Solid Edge part; units mm, degrees
sketch "Sketch1" plane through (0, 0, 0) normal (0, 0, 1) x (1, 0, 0)
  line L0 (8.65, -8) -> (-8.65, -8)
  line L1 (-8.65, -8) -> (-8.65, 8)
  line L2 (-8.65, 8) -> (8.65, 8)
  line L3 (8.65, 8) -> (8.65, -8)
  dimension "D1" = 8.65
  dimension "D2" = 8.65
extrude "Protrusion1" add sketch "Sketch1" along normal blind 6.5
sketch "Sketch2" plane through (0, 0, 6.5) normal (0, 0, 1) x (0, 1, 0)
  circle A0 centre (0, 0.35) radius 4.5
extrude "ExtrudedProtrusion_2" add sketch "Sketch2" along normal blind 7
sketch "Sketch3" plane through (0, 0, 6.5) normal (0, 0, 1) x (1, 0, 0)
  line L0 (8.65, 2) -> (12.15, 2)
  line L1 (12.15, 2) -> (12.15, -2)
  line L2 (12.15, -2) -> (8.65, -2)
  line L3 (8.65, -2) -> (8.65, 2)
  dimension "D1" = 12.15
extrude "ExtrudedProtrusion_3" add sketch "Sketch3" against normal blind 3
sketch "Sketch4" plane through (1.75, 0, 6.5) normal (0, 0, 1) x (1, 0, 0)
  arc A0 (6.9, 1.5) -> (6.9, -1.5) centre (6.9, 0) cw
  line L0 (6.9, 1.5) -> (6.9, -1.5)
extrude "ExtrudedProtrusion_4" add sketch "Sketch4" along normal blind 2
sketch "Sketch5" plane through (-0.35, 0, 13.5) normal (0, 0, 1) x (1, 0, 0)
  circle A0 centre (0, 0) radius 3
extrude "ExtrudedProtrusion_5" add sketch "Sketch5" along normal blind 13
Part model, mm, in its own coordinate system. A direction names the side the tool comes from. Give positions to 0.01 mm unless a question says otherwise; leave off trailing zeros. Order: outer loops, then holes, each group sorted by start corner. A loop starts at its lowest first (then second) coordinate and runs counter-clockwise, first axis right, second up. Notation, with made-up numbers: (88.5, 57.25) - (119.5, 57.25) arc R24 cw to (119.5, 75.25) - close; hole circle Ø11 at (-30, -33). An arc over 180 degrees is marked (long way). Use a Markdown table: item, result.
1) Saw through at B-B on z = 6. List the corners of the cut face in (x, y), plus the area to 3 significant figures.
Checked values:
| item | result |
|---|---|
| outline | (-8.65, -8) - (8.65, -8) - (8.65, -2) - (12.15, -2) - (12.15, 2) - (8.65, 2) - (8.65, 8) - (-8.65, 8) - close |
| area | 291 mm² |
2) Saw through at A-A on x = -0.35. List the corners of the cut face in (y, z), plus the area to 3 significant figures.
Checked values:
| item | result |
|---|---|
| outline | (-8, 0) - (8, 0) - (8, 6.5) - (4.5, 6.5) - (4.5, 13.5) - (3, 13.5) - (3, 26.5) - (-3, 26.5) - (-3, 13.5) - (-4.5, 13.5) - (-4.5, 6.5) - (-8, 6.5) - close |
| area | 245 mm² |
3) Probe L1, parallel to X at y = -4, z = 1.5; L2, parallel to Y at x = 11, z = 4; L3, parallel to Z at x = 0, y = 6.5. List the from-to ranges inside material, lowest first. Write a range as from..to.
Checked values:
| item | result |
|---|---|
| L1 | -8.65..8.65 |
| L2 | -2..2 |
| L3 | 0..6.5 |
4) 3-axis set-ups, long thin cutter, end or side, ignore diameter. For faces 1 (the cylindrical face through (10.15, 0.03, 7.49)), 2 (the cylindrical face through (-3.09, -3.57, 9.95)), 3 (the flat face through (10, 0, 3.5)), 4 (the flat face through (9, 0, 8.5)): which of +Z, -Z, +X, -X, +Y, -Y reach the whole face in a straight line?
Checked values:
| item | result |
|---|---|
| face 1 | +Z, +X |
| face 2 | +Z |
| face 3 | -Z, +X, +Y, -Y |
| face 4 | +Z, +X, +Y, -Y |
5) Flat gauge pins, fed straight in: P1, Ø3, axis at y = 3, z = 10.5, coming from the -X side; P2, Ø3.5, axis at x = 11, z = 5.5, coming from the -Y side; P3, Ø8, axis at y = -1, z = 15, coming from the -X side. Where does each tip first touch, or does it go through?
Checked values:
| item | result |
|---|---|
| P1 | x = -4.59 |
| P2 | y = -2 |
| P3 | x = -4.85 |
6) Saw through at C-C on y = 5. List the corners of the cut face in (x, z).
Checked values:
| item | result |
|---|---|
| outline | (-8.65, 0) - (8.65, 0) - (8.65, 6.5) - (-8.65, 6.5) - close |
7) Saw through at D-D on x = -4.25. List the corners of the cut face in (y, z) (3 decimals), plus the area to 3 significant figures.
Checked values:
| item | result |
|---|---|
| outline | (-8, 0) - (8, 0) - (8, 6.5) - (2.245, 6.5) - (2.245, 13.5) - (-2.245, 13.5) - (-2.245, 6.5) - (-8, 6.5) - close |
| area | 135 mm² |
8) Two-plate mould, pull along X, no slides. Class faces 5 (the cylindrical face through (2.51, -0.9, 19.91)), 6 (the flat face through (12.15, 0, 5)), 7 (the flat face through (10, -2, 5)), 8 (the flat face through (8.65, 0, 7)): +X half, -X half, draft (parallel to the pull), parting line (faces both ways), or undercut.
Checked values:
| item | result |
|---|---|
| face 5 | parting line |
| face 6 | +X half |
| face 7 | draft |
| face 8 | undercut |
